from build123d import *

# Parameters (mm, degrees)
SKETCH1_W                = 54.864
SKETCH1_H                = 28.194
SKETCH1_W_2              = 41.656
SKETCH1_H_2              = 21.59
BOSS_EXTRUDE1_DEPTH      = 3.175
BOSS_EXTRUDE2_DEPTH      = 6.096
BOSS_EXTRUDE2_DEPTH_BACK = 19.558
SKETCH1_3_W              = 41.656
SKETCH1_3_H              = 21.59
SKETCH1_3_W_2            = 34.29
SKETCH1_3_H_2            = 17.772256098


with BuildPart() as part:
    # Sketch1 → Boss-Extrude1 (new body)
    with BuildSketch(Plane(origin=(0, 0, 0), x_dir=(1, 0, 0), z_dir=(0, 1, 0))):
        with Locations((27.432, 14.097)):
            Rectangle(SKETCH1_W, SKETCH1_H)
        with Locations((27.432, 14.097)):
            Rectangle(SKETCH1_W_2, SKETCH1_H_2, mode=Mode.SUBTRACT)
    extrude(amount=BOSS_EXTRUDE1_DEPTH)

    # Sketch1<3> → Boss-Extrude2 (add, two sides: drawn at the far end of the back side and taken through both)
    with BuildSketch(Plane(origin=(0, 0, 0), x_dir=(1, 0, 0), z_dir=(0, 1, 0)).offset(-BOSS_EXTRUDE2_DEPTH_BACK)):
        with Locations((27.432, 14.097)):
            Rectangle(SKETCH1_3_W, SKETCH1_3_H)
        with Locations((27.432, 14.097)):
            Rectangle(SKETCH1_3_W_2, SKETCH1_3_H_2, mode=Mode.SUBTRACT)
    extrude(amount=BOSS_EXTRUDE2_DEPTH + BOSS_EXTRUDE2_DEPTH_BACK)


solid = part.part
Verification items for the finished model (mm, model axes). A direction names the side the tool comes from. Round coordinates to 2 decimals unless told otherwise and drop trailing zeros. Write each loop counter-clockwise with the first axis right and the second up, starting at its lowest first coordinate (ties: lowest second). Pieces come first, ordered by that corner, then holes.
(1) Depth check by flat-ended pin: pin 1 Ø3 at (y, z) = (-5, -16.5) entering from +X; pin 2 Ø2.5 at (x, y) = (36, 5) entering from +Z; pin 3 Ø14 at (x, z) = (28.5, -12.5) entering from -Y; pin 4 Ø6 at (x, y) = (24.5, -1) entering from -Z. Enter the tip coordinate at first touch or a pass-through.
Returned:
pin 1: stops at x = 48.26
pin 2: stops at z = -3.3
pin 3: passes through
pin 4: stops at z = -28.19
(2) Mould release check, pull along X, two halves, no side actions. Record for faces 5 (the flat face through (48.26, 5, -14)), 6 (the flat face through (6.604, 5, -14)), 7 (the flat face through (44.577, -7, -14)), 8 (the flat face through (27, -10, -24.892)): pulls with the +X half, pulls with the -X half, needs draft (parallel to the pull), parting line crosses it, or undercut.
Returned:
face 5: pulls with the +X half
face 6: pulls with the -X half
face 7: undercut
face 8: needs draft
(3) Section check D-D (y = -8). Enter the section's corners in (x, z).
Returned:
outline: (6.6, -24.89) - (48.26, -24.89) - (48.26, -3.3) - (6.6, -3.3) - close; hole (10.29, -22.98) - (44.58, -22.98) - (44.58, -5.21) - (10.29, -5.21) - close
(4) Section check C-C (z = -8.75). Enter the section's corners in (x, y) (3 decimals).
Returned:
outline: (0, 0) - (6.604, 0) - (6.604, -19.558) - (10.287, -19.558) - (10.287, 6.096) - (6.604, 6.096) - (6.604, 3.175) - (0, 3.175) - close; (44.577, -19.558) - (48.26, -19.558) - (48.26, 0) - (54.864, 0) - (54.864, 3.175) - (48.26, 3.175) - (48.26, 6.096) - (44.577, 6.096) - close
(5) Section check A-A (y = 1). Enter the section's corners in (x, z), plus the area to 3 significant figures.
Returned:
outline: (0, -28.19) - (54.86, -28.19) - (54.86, 0) - (0, 0) - close; hole (10.29, -22.98) - (44.58, -22.98) - (44.58, -5.21) - (10.29, -5.21) - close
area: 937 mm2
(6) Access from +Z, -Z, +X, -X, +Y, -Y to the whole of each face (thin tool, end or side, straight path). Record for faces 1 (the flat face through (27, 5, -24.892)), 2 (the flat face through (10.287, -7, -14)), 3 (the flat face through (27, -10, -3.302)), 4 (the flat face through (48.26, -10, -14)).
Returned:
face 1: -Z, +X, -X, +Y
face 2: +Y, -Y
face 3: +Z, +X, -X, -Y
face 4: +Z, -Z, +X, -Y
(7) Section check B-B (x = 30.5). Enter the section's corners in (y, z) (3 decimals), plus the area to 3 significant figures.
Returned:
outline: (-19.558, -24.892) - (0, -24.892) - (0, -28.194) - (3.175, -28.194) - (3.175, -24.892) - (6.096, -24.892) - (6.096, -22.983) - (-19.558, -22.983) - close; (-19.558, -5.211) - (6.096, -5.211) - (6.096, -3.302) - (3.175, -3.302) - (3.175, 0) - (0, 0) - (0, -3.302) - (-19.558, -3.302) - close
area: 119 mm2
(8) Material ranges on line 1 (X direction, y = -0.5, z = -7.5); line 2 (Z direction, x = 22.5, y = -1); line 3 (Z direction, x = 7, y = -2.5), recorded low to high.
Returned:
line 1: x = 6.6 to 10.29, 44.58 to 48.26
line 2: z = -24.89 to -22.98, -5.21 to -3.3
line 3: z = -24.89 to -3.3
